The listing builds one solid part. Answer for the finished solid, in the listing's coordinates (mm). A direction names the side the tool comes from. Give positions to 0.01 mm unless a question says otherwise; leave off trailing zeros. Write each loop counter-clockwise with the first axis right and the second up, starting at its lowest first coordinate (ties: lowest second). Pieces come first, ordered by that corner, then holes. Notation, with made-up numbers: M 10,37.25 L 27,37.25 A28 ccw 27,68.25 Z; hole C 11,89.5 d1. An arc over 180 degrees is marked long. Answer as a JSON object with one key per item and string values.
```python
from build123d import *

# Parameters (mm, degrees)
SKETCH1_W               = 50.8
SKETCH1_H               = 50.8
BASE_FLANGE1_DEPTH      = 0.7
EDGE_FLANGE1_DEPTH      = 50.8
EDGE_FLANGE1_BEND_DEPTH = 50.8
SKETCH12_R              = 3.5
CUT_EXTRUDE1_DEPTH      = 45.605605029
SKETCH13_R              = 1
CUT_EXTRUDE2_DEPTH      = 45.605605029
SKETCH14_R              = 1.6
CUT_EXTRUDE3_DEPTH      = 65.752528908


# Sheet-metal steps are written as plain solids
with BuildPart() as part:
    # Sketch1 → Base-Flange1 (new body)
    with BuildSketch(Plane(origin=(0, 0, 0), x_dir=(1, 0, 0), z_dir=(0, 1, 0))):
        Rectangle(SKETCH1_W, SKETCH1_H)
    extrude(amount=-BASE_FLANGE1_DEPTH)

    # Edge-Flange1 section (across the edge) → Edge-Flange1 (add)
    with BuildSketch(Plane(origin=(25.4, 0, -26.4), x_dir=(0, 0, 1), z_dir=(-1, 0, 0))):
        with BuildLine():
            Line((-0.7, 1), (-0.7, 24.7))
            Line((-0.7, 24.7), (0, 24.7))
            Line((0, 24.7), (0, 1))
            ThreePointArc((0, 1), (0.292893219, 0.292893219), (1, 0))
            Line((1, 0), (1, -0.7))
            ThreePointArc((1, -0.7), (-0.202081528, -0.202081528), (-0.7, 1))
        make_face()
    extrude(amount=EDGE_FLANGE1_DEPTH)

    # Edge-Flange1 section 2 (across the edge) → Edge-Flange1 bend (add)
    with BuildSketch(Plane(origin=(-25.4, 0, 26.4), x_dir=(0, 0, -1), z_dir=(1, 0, 0))):
        with BuildLine():
            Line((-0.7, 1), (-0.7, 24.7))
            Line((-0.7, 24.7), (0, 24.7))
            Line((0, 24.7), (0, 1))
            ThreePointArc((0, 1), (0.292893219, 0.292893219), (1, 0))
            Line((1, 0), (1, -0.7))
            ThreePointArc((1, -0.7), (-0.202081528, -0.202081528), (-0.7, 1))
        make_face()
    extrude(amount=EDGE_FLANGE1_BEND_DEPTH)

    # Sketch12 → Cut-Extrude1 (cut, through all)
    with BuildSketch(Plane(origin=(0, 0, 0), x_dir=(1, 0, 0), z_dir=(0, 1, 0))):
        with Locations(Location((20.4, -20.4, 0), (0, 0, 270))):
            Circle(SKETCH12_R)
    extrude(amount=-CUT_EXTRUDE1_DEPTH, mode=Mode.SUBTRACT)

    # Sketch13 → Cut-Extrude2 (cut, through all)
    with BuildSketch(Plane(origin=(0, 0, 0), x_dir=(1, 0, 0), z_dir=(0, 1, 0))):
        with Locations(Location((1.4, -20.4, 0), (0, 0, 270))):
            Circle(SKETCH13_R)
    extrude(amount=-CUT_EXTRUDE2_DEPTH, mode=Mode.SUBTRACT)

    # Sketch14 → Cut-Extrude3 (cut, through all)
    with BuildSketch(Plane.XY.offset(27.1)):
        with Locations((0, 19.7)):
            Circle(SKETCH14_R)
    extrude(amount=-CUT_EXTRUDE3_DEPTH, mode=Mode.SUBTRACT)


solid = part.part
```
1. Consider line 1 along X through (y, z) = (-0.4, 20.4); line 2 along Z through (x, y) = (-3.5, 7); line 3 along Y through (x, z) = (11, -18.5). Determine where each line is inside the solid, lowest interval first.
Verdict:
{"line 1": "x = -25.4 to 0.4, 2.4 to 16.9, 23.9 to 25.4", "line 2": "z = -27.1 to -26.4, 26.4 to 27.1", "line 3": "y = -0.7 to 0"}
2. A cutting plane is placed at B-B, the plane z = 20.4. Give the vertices of the cut face in (x, y), plus the area to 3 significant figures.
Verdict:
{"outline": "M -25.4,-0.7 L 0.4,-0.7 L 0.4,0 L -25.4,0 Z; M 2.4,-0.7 L 16.9,-0.7 L 16.9,0 L 2.4,0 Z; M 23.9,-0.7 L 25.4,-0.7 L 25.4,0 L 23.9,0 Z", "area": "29.3 mm2"}
3. The mould has two halves that part along Y. Classify faces 1 (the cylindrical face through (-0.35, 18.14, -26.75)), 2 (the flat face through (0, 0, 0)), 3 (the flat face through (0, 13, -27.1)): released by +Y, released by -Y, zero draft, split by the parting line, or undercut.
Verdict:
{"face 1": "undercut", "face 2": "released by +Y", "face 3": "zero draft"}
4. A cutting plane is placed at D-D, the plane x = -9.5. Give the vertices of the cut face in (y, z), plus the area to 3 significant figures.
Verdict:
{"outline": "M -0.7,-25.4 A1.7 ccw 1,-27.1 L 24.7,-27.1 L 24.7,-26.4 L 1,-26.4 A1 cw 0,-25.4 L 0,25.4 A1 cw 1,26.4 L 24.7,26.4 L 24.7,27.1 L 1,27.1 A1.7 ccw -0.7,25.4 Z", "area": "71.7 mm2"}
5. A cutting plane is placed at A-A, the plane x = 20.4. Give the vertices of the cut face in (y, z), plus the area to 3 significant figures.
Verdict:
{"outline": "M -0.7,-25.4 A1.7 ccw 1,-27.1 L 24.7,-27.1 L 24.7,-26.4 L 1,-26.4 A1 cw 0,-25.4 L 0,16.9 L -0.7,16.9 Z; M -0.7,23.9 L 0,23.9 L 0,25.4 A1 cw 1,26.4 L 24.7,26.4 L 24.7,27.1 L 1,27.1 A1.7 ccw -0.7,25.4 Z", "area": "66.8 mm2"}
6. A cutting plane is placed at C-C, the plane y = 14.25. Give the vertices of the cut face in (x, z).
Verdict:
{"outline": "M -25.4,-27.1 L 25.4,-27.1 L 25.4,-26.4 L -25.4,-26.4 Z; M -25.4,26.4 L 25.4,26.4 L 25.4,27.1 L -25.4,27.1 Z"}
7. For faces 4 (the cylindrical face through (-0.35, 18.14, 26.75)), 5 (the flat face through (0, 13, 26.4)), determine the directions among +Z, -Z, +X, -X, +Y, -Y from which every point of the face is accessible in a straight line to the end or side of a thin tool.
Verdict:
{"face 4": "+Z, -Z", "face 5": "+X, -X, +Y"}
8. Flat-ended cylindrical pins translate along their axes: pin 1 (1.5 mm diameter, centred on x = -18.5, z = 20, fed in from +Y); pin 2 (10 mm diameter, centred on y = 16.5, z = -17.5, fed in from -X). Find the tip coordinate at first contact, or state that the pin passes through.
Verdict:
{"pin 1": "stops at y = 0", "pin 2": "passes through"}
